Build history of the part. All positions in model axes, mm. A direction names the side the tool comes from. Round coordinates to 2 decimals unless told otherwise and drop trailing zeros. Order: outer loops, then holes, each group sorted by start corner. A loop starts at its lowest first (then second) coordinate and runs counter-clockwise, first axis right, second up. Notation, with made-up numbers: M -24.5,24.5 L -4.5,24.5 A18 ccw -4.5,59.5 Z; hole C 51.5,47.5 d7. An arc over 180 degrees is marked long. Use CSV: the item, a comma, the result in double quotes.
from build123d import *

# Parameters (mm, degrees)
F0_R     = 15
F1_DEPTH = 55
F2_R     = 15
F3_DEPTH = 26
F4_R     = 10.85
F5_DEPTH = 55
F6_R     = 10.85
F7_DEPTH = 26


with BuildPart() as f1:
    # F0 (on Top) → F1 (new body)
    with BuildSketch(Plane.XY):
        Circle(F0_R)
    extrude(amount=F1_DEPTH)

    # F2 (on Front) → F3 (join)
    with BuildSketch(Plane.XZ):
        with Locations((0, 27.5)):
            Circle(F2_R)
    extrude(amount=F3_DEPTH)

    # F4 (on face) → F5 (cut)
    with BuildSketch(Plane.XY.offset(55)):
        Circle(F4_R)
    extrude(amount=-F5_DEPTH, mode=Mode.SUBTRACT)

    # F6 (on face) → F7 (cut)
    with BuildSketch(Plane.XZ.offset(26)):
        with Locations((0, 27.5)):
            Circle(F6_R)
    extrude(amount=-F7_DEPTH, mode=Mode.SUBTRACT)


solid = f1.part
(1) Tool access for faces 5 (the face through (-14.985, -15.707, 28.16)), 6 (the face through (-1.953, 14.872, 27.115)), 7 (the face through (7.71, -26, 35.35)): list every direction of +Z, -Z, +X, -X, +Y, -Y with a clear straight run to the whole face (end or side of a thin tool).
Answer block:
face 5,"-Y"
face 6,"none"
face 7,"+Z, -Z, +X, -X, -Y"
(2) Two-plate mould, pull along Z, no slides. Class faces 1 (the face through (10, 5, 55)), 2 (the face through (10, 5, 0)), 3 (the face through (-10.84, -16.07, 27.98)), 4 (the face through (-1.41, 10.76, 27.88)): released by +Z, released by -Z, zero draft, split by the parting line, or undercut.
Answer block:
face 1,"released by +Z"
face 2,"released by -Z"
face 3,"undercut"
face 4,"zero draft"
(3) Cut at A-A, the plane x = 0. Give the cut face in (y, z), and give its area (3 significant figures).
Answer block:
outline,"M -26,12.5 L -15,12.5 L -15,0 L -10.85,0 L -10.85,16.65 L -26,16.65 Z; M -26,38.35 L -10.85,38.35 L -10.85,55 L -15,55 L -15,42.5 L -26,42.5 Z; M 10.85,0 L 15,0 L 15,55 L 10.85,55 Z"
area,"458 mm²"
(4) Drop flat-ended pins along their axis: pin 1 (8 mm diameter, centred on x = -1, z = 24.5, fed in from -Y); pin 2 (4 mm diameter, centred on x = 4.5, z = 13.5, fed in from +Y); pin 3 (1.5 mm diameter, centred on x = 1, z = 44.5, fed in from -Y). Give the stop position or say it passes through.
Answer block:
pin 1,"stops at y = 9.63"
pin 2,"stops at y = 14.79"
pin 3,"stops at y = -15"
(5) Cut at C-C, the plane z = 27.5. Give the cut face in (x, y), and give its area (3 significant figures).
Answer block:
outline,"M -15,-26 L -10.85,-26 L -10.85,0 A10.85 cw 10.85,0 L 10.85,-26 L 15,-26 L 15,0 A15 ccw -15,0 Z"
area,"384 mm²"
(6) Cut at D-D, the plane z = 5. Give the cut face in (x, y).
Answer block:
outline,"C 0,0 d30; hole C 0,0 d21.7"
(7) Cut at B-B, the plane y = 7. Give the cut face in (x, z).
Answer block:
outline,"M -13.27,0 L -8.29,0 L -8.29,55 L -13.27,55 Z; M 8.29,0 L 13.27,0 L 13.27,55 L 8.29,55 Z"
(8) Wall check: line 1 (X direction, y = -7, z = 27); line 2 (Z direction, x = -0.5, y = -16); line 3 (Z direction, x = -4.75, y = -11.5) (3 decimals). Give the ranges that are in metal, low to high. Write a range as from..to.
Answer block:
line 1,"x = -14.99..-10.84, 10.84..14.99"
line 2,"z = 12.51..16.66, 38.34..42.49"
line 3,"z = 0..17.745, 37.255..55"
